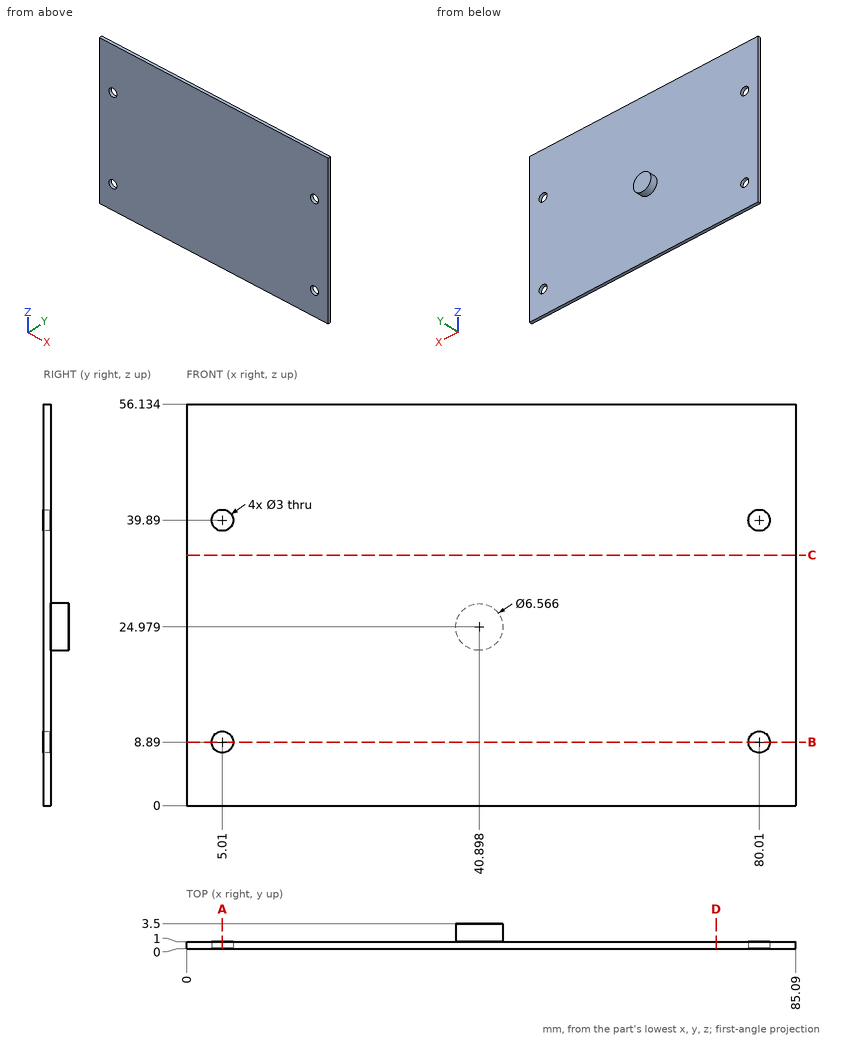
Can you work these out from the drawing? Everything is in mm from the part's minimum corner. Round coordinates to 2 decimals unless told otherwise and drop trailing zeros. Loops run counter-clockwise (first coordinate to the right, second up) from the corner with the lowest first, then second, coordinate; pieces in that order, holes last. Notation, with made-up numbers: (27.25, -17.75) - (76.25, -17.75) arc R28 cw to (76.25, 16.25) - close; hole circle Ø3 at (87, 53.25). An arc over 180 degrees is marked (long way). One line per question, with ' | ' between items. Start each with the question number.
Q1. I want a section at B-B (z = 8.89). Write out the boundary of the cut face in (x, y).
Q2. I want a section at C-C (z = 35). Write out the boundary of the cut face in (x, y).
Q3. I want a section at A-A (x = 5.01). Write out the boundary of the cut face in (y, z).
Q4. Will these pins go through, and if not, where does the flat tip stop? pin 1 (6 mm diameter, centred on x = 75.5, z = 7, fed in from +Y); pin 2 (1.5 mm diameter, centred on y = 3, z = 47, fed in from +X).
Q5. Please list where these lines run through material, in increasing order: line 1 (Y direction, x = 30.5, z = 14); line 2 (Z direction, x = 43.5, y = 2.5) (1 decimal). Write a range as [from, to].
Q6. I want a section at D-D (x = 74). Write out the boundary of the cut face in (y, z).
Response values:
1) outline: (0, 0) - (3.51, 0) - (3.51, 1) - (0, 1) - close; (6.51, 0) - (78.51, 0) - (78.51, 1) - (6.51, 1) - close; (81.51, 0) - (85.09, 0) - (85.09, 1) - (81.51, 1) - close
2) outline: (0, 0) - (85.09, 0) - (85.09, 1) - (0, 1) - close
3) outline: (0, 0) - (1, 0) - (1, 7.39) - (0, 7.39) - close; (0, 10.39) - (1, 10.39) - (1, 38.39) - (0, 38.39) - close; (0, 41.39) - (1, 41.39) - (1, 56.13) - (0, 56.13) - close
4) pin 1: stops at y = 1 | pin 2: passes through
5) line 1: y = [0, 1] | line 2: z = [23, 27]
6) outline: (0, 0) - (1, 0) - (1, 56.13) - (0, 56.13) - close
